The model under review builds one solid part; all positions refer to its coordinate system, in mm. A direction names the side the tool comes from. Round coordinates to 2 decimals unless told otherwise and drop trailing zeros. Write each loop counter-clockwise with the first axis right and the second up, starting at its lowest first coordinate (ties: lowest second). Pieces come first, ordered by that corner, then holes. Notation, with made-up numbers: M 1.25,10 L 45.25,10 A3 cw 45.25,14 Z; hole C -28.75,45 d8. An arc over 180 degrees is marked long. One line per item, written item: value. Start each with the question number.
1) Take a section at A-A, the plane y = -9.65. Write out the cut boundary in (x, z), and give its area (3 significant figures).
2) Mouldability with a two-part tool opening along X and no side actions: class faces 1 (the face through (-49, -20, 1)), 2 (the face through (1, 19, 1)), 3 (the face through (18.66, 4.66, 1.48)) as +X half, -X half, draft (parallel to the pull), parting line (faces both ways), or undercut.
3) Take a section at D-D, the plane x = -35.9. Write out the cut boundary in (y, z), and give its area (3 significant figures).
4) For P1, Ø0.9, axis at x = -47, z = 1, coming from the +Y side; P2, Ø1.2, axis at y = -20.5, z = 2, coming from the -X side; P3, Ø1.5, axis at y = -13, z = 1, coming from the -X side, all flat-tipped, find the tip position at first contact; note any pin that passes through.
5) Take a section at C-C, the plane y = 6.8. Write out the cut boundary in (x, z) (3 decimals), and give its area (4 significant figures).
6) Tool access review of faces 4 (the face through (-1, -19, 1)), 5 (the face through (49, -20, 1)), 6 (the face through (53, 5, 1)): name each direction out of +Z, -Z, +X, -X, +Y, -Y from which nothing blocks a thin tool from reaching the whole face with its end or side.
7) Take a section at B-B, the plane x = 6.43. Write out the cut boundary in (y, z), and give its area (3 significant figures).
8) Wall thickness on probe 1 along X at (y, z) = (7, 0.25); probe 2 along Y at (x, z) = (6.43, 1.45); probe 3 along Y at (x, z) = (18, 2.25): over which ranges is each line inside the solid? List them lowest first.
from build123d import *

# Parameters (mm, degrees)
SKETCH_1_R      = 3.1
SKETCH_1_R_2    = 3.35
SKETCH_1_R_3    = 3.6
SKETCH_1_R_4    = 3.85
SKETCH_1_R_5    = 4.1
SKETCH_1_R_6    = 4.35
SKETCH_1_R_7    = 4.6
SKETCH_1_R_8    = 4.85
SKETCH_1_R_9    = 5.1
SKETCH_1_R_10   = 5.6
SKETCH_1_R_11   = 6.1
SKETCH_1_W      = 3
SKETCH_1_H      = 10
EXTRUDE_1_DEPTH = 3
FILLET_1_R      = 0.5
FILLET_2_R      = 1


with BuildPart() as part:
    # Эскиз1 → Бобышка-Вытянуть1 (new body)
    with BuildSketch(Plane.XY):
        Polygon((39, 19), (-39, 19), (-39, 16), (-52, 16), (-52, 5), (-52, -5), (-52, -19), (-49, -19), (-49, -22), (-46, -22), (-46, -19), (0, -19), (46, -19), (46, -22), (49, -22), (49, -19), (52, -19), (52, -5), (52, 5), (52, 16), (39, 16), align=None)
        with Locations((-35.9, -9.65)):
            Circle(SKETCH_1_R, mode=Mode.SUBTRACT)
        with Locations((-21.79, -9.65)):
            Circle(SKETCH_1_R_2, mode=Mode.SUBTRACT)
        with Locations((-7.68, -9.65)):
            Circle(SKETCH_1_R_3, mode=Mode.SUBTRACT)
        with Locations((6.43, -9.65)):
            Circle(SKETCH_1_R_4, mode=Mode.SUBTRACT)
        with Locations((20.54, -9.65)):
            Circle(SKETCH_1_R_5, mode=Mode.SUBTRACT)
        with Locations((34.65, -9.65)):
            Circle(SKETCH_1_R_6, mode=Mode.SUBTRACT)
        with Locations((-28.845, 6.8)):
            Circle(SKETCH_1_R_7, mode=Mode.SUBTRACT)
        with Locations((-14.735, 6.8)):
            Circle(SKETCH_1_R_8, mode=Mode.SUBTRACT)
        with Locations((-0.625, 6.8)):
            Circle(SKETCH_1_R_9, mode=Mode.SUBTRACT)
        with Locations((13.485, 6.8)):
            Circle(SKETCH_1_R_10, mode=Mode.SUBTRACT)
        with Locations((27.595, 6.8)):
            Circle(SKETCH_1_R_11, mode=Mode.SUBTRACT)
        with Locations((-53.5, 0)):
            Rectangle(SKETCH_1_W, SKETCH_1_H)
        with Locations((53.5, 0)):
            Rectangle(SKETCH_1_W, SKETCH_1_H)
    extrude(amount=EXTRUDE_1_DEPTH)

    # Скругление1
    fillet_1_edges = [part.edges().sort_by_distance(p)[0] for p in [
        (-55, -5, 1.5),
        (-55, 5, 1.5),
        (55, 5, 1.5),
        (55, -5, 1.5),
        (49, -22, 1.5),
        (46, -22, 1.5),
        (-46, -22, 1.5),
        (-49, -22, 1.5),
    ]]
    fillet(fillet_1_edges, radius=FILLET_1_R)

    # Скругление2
    fillet_2_edges = [part.edges().sort_by_distance(p)[0] for p in [
        (-52, -19, 1.5),
        (-52, 16, 1.5),
        (-39, 16, 1.5),
        (-39, 19, 1.5),
        (39, 19, 1.5),
        (39, 16, 1.5),
        (52, 16, 1.5),
        (52, -19, 1.5),
    ]]
    fillet(fillet_2_edges, radius=FILLET_2_R)


solid = part.part
Checked values:
1. outline: M -52,0 L -39,0 L -39,3 L -52,3 Z; M -32.8,0 L -25.14,0 L -25.14,3 L -32.8,3 Z; M -18.44,0 L -11.28,0 L -11.28,3 L -18.44,3 Z; M -4.08,0 L 2.58,0 L 2.58,3 L -4.08,3 Z; M 10.28,0 L 16.44,0 L 16.44,3 L 10.28,3 Z; M 24.64,0 L 30.3,0 L 30.3,3 L 24.64,3 Z; M 39,0 L 52,0 L 52,3 L 39,3 Z
1. area: 178 mm2
2. face 1: -X half
2. face 2: draft
2. face 3: undercut
3. outline: M -19,0 L -12.75,0 L -12.75,3 L -19,3 Z; M -6.55,0 L 19,0 L 19,3 L -6.55,3 Z
3. area: 95.4 mm2
4. P1: stops at y = 16
4. P2: stops at x = -49
4. P3: stops at x = -52
5. outline: M -52,0 L -33.445,0 L -33.445,3 L -52,3 Z; M -24.245,0 L -19.585,0 L -19.585,3 L -24.245,3 Z; M -9.885,0 L -5.725,0 L -5.725,3 L -9.885,3 Z; M 4.475,0 L 7.885,0 L 7.885,3 L 4.475,3 Z; M 19.085,0 L 21.495,0 L 21.495,3 L 19.085,3 Z; M 33.695,0 L 52,0 L 52,3 L 33.695,3 Z
5. area: 154.5 mm2
6. face 4: +Z, -Z, -Y
6. face 5: +Z, -Z, +X, -Y
6. face 6: +Z, -Z, +X, +Y
7. outline: M -19,0 L -13.5,0 L -13.5,3 L -19,3 Z; M -5.8,0 L 19,0 L 19,3 L -5.8,3 Z
7. area: 90.9 mm2
8. probe 1: x = -52 to -33.44, -24.25 to -19.58, -9.89 to -5.72, 4.47 to 7.89, 19.08 to 21.5, 33.69 to 52
8. probe 2: y = -19 to -13.5, -5.8 to 19
8. probe 3: y = -19 to -12.87, -6.43 to 3.49, 10.11 to 19
